The drawing under review shows one solid part. Ordinate dimensions are in mm from its lowest x, y, z. A direction names the side the tool comes from. Round coordinates to 2 decimals unless told otherwise and drop trailing zeros. Write each loop counter-clockwise with the first axis right and the second up, starting at its lowest first coordinate (ties: lowest second). Pieces come first, ordered by that corner, then holes. Notation, with made-up numbers: M -2.75,-10.75 L 50.25,-10.75 A20 ccw 50.25,18.25 Z; hole C 44,49.5 d11. An arc over 180 degrees is marked long. Write item = value, one per line. Start each with the question number.
Item 1: Take a section at C-C, the plane z = 57.5. Give the boundary of the cut face in (x, y).
Item 2: Take a section at A-A, the plane x = 50.8. Give the boundary of the cut face in (y, z).
Item 3: Take a section at B-B, the plane y = 18.85. Give the boundary of the cut face in (x, z).
Item 4: The part is to be moulded in two halves that separate along Z. For the marked faces 6, 7 and 8, say which applies: +Z half, -Z half, draft (parallel to the pull), parting line (faces both ways), or undercut.
Item 5: To check wall thickness, follow line 1 along Z through (x, y) = (133, 25.5); line 2 along X through (y, z) = (18.85, 76); line 3 along Y through (x, z) = (63.5, 14.5). State the ranges of each line that lie inside material, in increasing order.
Item 6: For pin 1 Ø10 at (y, z) = (24, 75.5) entering from -X; pin 2 Ø12 at (x, z) = (93, 51) entering from +Y; pin 3 Ø12.5 at (x, y) = (108, 20.5) entering from -Z, all flat-tipped, find the tip position at first contact; note any pin that passes through.
Item 7: Tool access review of the marked faces 1, 2, 3, 4 and 5: name each direction out of +Z, -Z, +X, -X, +Y, -Y from which nothing blocks a thin tool from reaching the whole face with its end or side.
Item 8: Take a section at D-D, the plane y = 26. Give the boundary of the cut face in (x, z).
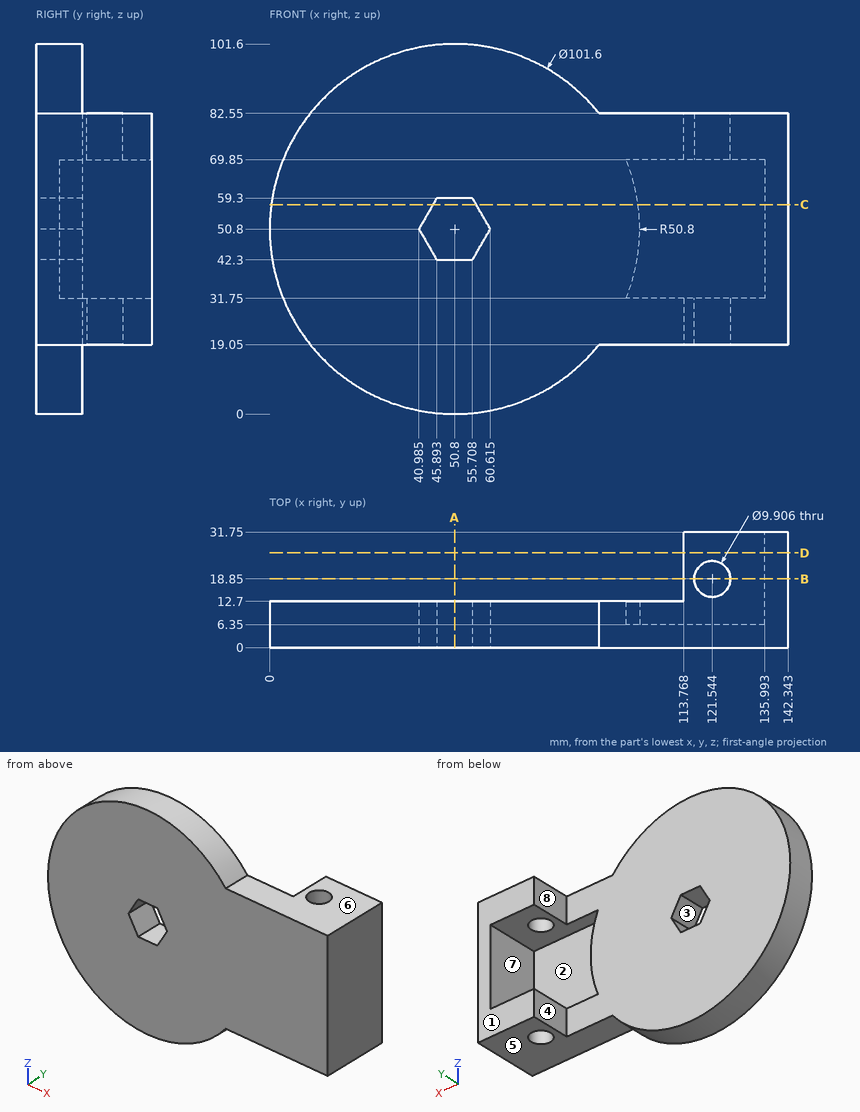
Response values:
q1.outline = M 0.44,0 L 44.85,0 L 44.85,12.7 L 0.44,12.7 Z; M 56.75,0 L 142.34,0 L 142.34,31.75 L 135.99,31.75 L 135.99,6.35 L 101.16,6.35 L 101.16,12.7 L 56.75,12.7 Z
q2.outline = M 0,0 L 12.7,0 L 12.7,42.3 L 0,42.3 Z; M 0,59.3 L 12.7,59.3 L 12.7,101.6 L 0,101.6 Z
q3.outline = M 113.77,19.05 L 116.59,19.05 L 116.59,31.75 L 113.77,31.75 Z; M 113.77,69.85 L 116.59,69.85 L 116.59,82.55 L 113.77,82.55 Z; M 126.5,19.05 L 142.34,19.05 L 142.34,82.55 L 126.5,82.55 L 126.5,69.85 L 135.99,69.85 L 135.99,31.75 L 126.5,31.75 Z
q4.face_6 = +Z half
q4.face_7 = undercut
q4.face_8 = draft
q5.line_1 = 19.05 to 31.75, 69.85 to 82.55
q5.line_2 = 113.77 to 116.59, 126.5 to 142.34
q5.line_3 = 0 to 12.7
q6.pin_1 = 113.77
q6.pin_2 = 12.7
q6.pin_3 = 19.05
q7.face_1 = +Z, -Z, +X, -X, +Y
q7.face_2 = +Y
q7.face_3 = +Y, -Y
q7.face_4 = +Z, -Z, -X, +Y
q7.face_5 = -Z, +X, +Y, -Y
q8.outline = M 113.77,19.05 L 142.34,19.05 L 142.34,82.55 L 113.77,82.55 L 113.77,69.85 L 135.99,69.85 L 135.99,31.75 L 113.77,31.75 Z
